Geometry check sheet. Reference: the model listing, model coordinates, mm. A direction names the side the tool comes from. Round coordinates to 2 decimals unless told otherwise and drop trailing zeros. Write each loop counter-clockwise with the first axis right and the second up, starting at its lowest first coordinate (ties: lowest second). Pieces come first, ordered by that corner, then holes. Notation, with made-up numbers: M 88.5,44.5 L 147.5,44.5 A19 ccw 147.5,68.5 Z; hole C 56,-10 d1. An arc over 180 degrees is marked long. One line per item, written item: value. Start each with the question number.
1. Depth check by flat-ended pin: P1, Ø6, axis at x = 50.5, y = -52, coming from the +Z side; P2, Ø10, axis at x = 45, y = -67.5, coming from the +Z side; P3, Ø8, axis at x = 19.5, y = -80.5, coming from the +Z side; P4, Ø8, axis at y = -20.5, z = 8, coming from the +X side. Enter the tip coordinate at first touch or a pass-through.
2. Scan lines: probe 1 along Z at (x, y) = (54, -25); probe 2 along X at (y, z) = (-89, 3); probe 3 along X at (y, z) = (-67, 25). Record each from-to range of solid material in increasing order. Write a range as [from, to].
3. Section check B-B (z = 28). Count the separate pieces of the cut face and the enclosed holes in it, and give its area (3 significant figures).
4. Access from +Z, -Z, +X, -X, +Y, -Y to the whole of each face (thin tool, end or side, straight path). Record for faces 1 (the flat face through (25, -72, 9)), 2 (the flat face through (75, -72, 9)), 3 (the flat face through (0, -49, -13)), 4 (the flat face through (50, -54, 0)), 5 (the flat face through (60, -27, 0)).
5. Section check C-C (y = -7). Record the boundary of the cut face in (x, z).
6. Release check for a two-part mould opening along Z. For faces 6 (the flat face through (100, -49, -13)), 7 (the flat face through (52.6, -67.9, 35.8)), 8 (the flat face through (49, -49, -25)), 9 (the cylindrical face through (40.787, -61.717, 30.587)) record: pulls with the +Z half, pulls with the -Z half, needs draft (parallel to the pull), parting line crosses it, or undercut.
7. Section check A-A (x = 52). Record the boundary of the cut face in (y, z), and give its area (3 significant figures).
8. Section check D-D (x = 22). Record the boundary of the cut face in (y, z), and give its area (3 significant figures).
from build123d import *

# Parameters (mm, degrees)
F0_W      = 100
F0_H      = 25
F1_DEPTH  = 100
F7_W      = 50
F7_H      = 40
F8_R      = 25
F9_R      = 12.5
F12_DEPTH = 15
F13_R     = 6
F14_REACH = 55.0172779755


with BuildPart() as f1:
    # F0 (on Front) → F1 (new body)
    with BuildSketch(Plane.XZ):
        with Locations((50, -12.5)):
            Rectangle(F0_W, F0_H)
    extrude(amount=F1_DEPTH)

    # F7 (on line) + F8 (on line) → F11 (join, up to the next surface of F1)
    with BuildSketch(Plane(origin=(0, -24.9763522297, 43.2603110496), x_dir=(1, 0, 0), z_dir=(0, -0.5, 0.8660254038))):
        with Locations((50, -66.6025403784)):
            Rectangle(F7_W, F7_H)
    with BuildSketch(Plane(origin=(0, -24.9763522297, 43.2603110496), x_dir=(1, 0, 0), z_dir=(0, -0.5, 0.8660254038))):
        with Locations((50, -46.6025403784)):
            Circle(F8_R)
    extrude(until=Until.NEXT, dir=(0, 0.5, -0.8660254038))

    # F9 (on line) → F12 (join)
    with BuildSketch(Plane(origin=(0, -24.9763522297, 43.2603110496), x_dir=(1, 0, 0), z_dir=(0, -0.5, 0.8660254038))):
        with Locations((50, -46.6025403784)):
            Circle(F9_R)
    extrude(amount=F12_DEPTH)

    f14_end = Plane.XY
    # F13 (on face) → F14 (cut, up to a plane its end follows)
    with BuildSketch(Plane(origin=(0, -32.4763522297, 56.2506921064), x_dir=(1, 0, 0), z_dir=(0, -0.5, 0.8660254038))):
        with Locations((50, -46.6025403784)):
            Circle(F13_R)
    f14_long = extrude(amount=-F14_REACH, mode=Mode.PRIVATE)
    add(split(f14_long, bisect_by=f14_end, keep=Keep.TOP, mode=Mode.PRIVATE), mode=Mode.SUBTRACT)


solid = f1.part
Result sheet:
1. P1: stops at z = 29.39
1. P2: stops at z = 38.86
1. P3: stops at z = 0
1. P4: passes through
2. probe 1: z = [-25, 0]
2. probe 2: x = [25, 75]
2. probe 3: x = [37.55, 44.1], [55.9, 62.45]
3. separate pieces: 2
3. enclosed holes: 1
3. area: 679 mm2
4. face 1: +Z, -X, +Y, -Y
4. face 2: +Z, +X, +Y, -Y
4. face 3: +Z, -Z, -X, +Y, -Y
4. face 4: none
4. face 5: +Z, +Y
5. outline: M 0,-25 L 100,-25 L 100,0 L 0,0 Z
6. face 6: needs draft
6. face 7: pulls with the +Z half
6. face 8: pulls with the -Z half
6. face 9: undercut
7. outline: M -100,-25 L 0,-25 L 0,0 L -25.04,0 L -43.75,32.42 L -54.65,26.13 L -62.15,39.12 L -67.94,35.78 L -47.28,0 L -60.34,0 L -77.73,30.12 L -83.52,26.78 L -76.02,13.79 L -99.91,0 L -100,0 Z
7. area: 3,650 mm2
8. outline: M -100,-25 L 0,-25 L 0,0 L -100,0 Z
8. area: 2,500 mm2
